from build123d import *

# Parameters (mm, degrees)
SKETCH1_W                                       = 50
SKETCH1_H                                       = 7.5
BOSS_EXTRUDE1_DEPTH                             = 5
FILLET1_R                                       = 2
SKETCH2_R                                       = 2.5
BOSS_EXTRUDE2_DEPTH                             = 3
CBORE_FOR_M3_SHCS1_D                            = 5.25
CBORE_FOR_M3_SHCS1_DEPTH                        = 4
CBORE_FOR_M3_SHCS1_CBORE_D                      = 6
CBORE_FOR_M3_SHCS1_CBORE_DEPTH                  = 0.5
CBORE_FOR_M3_SHCS1_TIP                          = 1.577259125
CSK_FOR_M3_FLAT_HEAD_MACHINE_SCREW1_D           = 3.4
CSK_FOR_M3_FLAT_HEAD_MACHINE_SCREW1_CSINK_D     = 6.3
CSK_FOR_M3_FLAT_HEAD_MACHINE_SCREW1_CSINK_ANGLE = 90
M3_CLEARANCE_HOLE1_D                            = 3.25
M3_CLEARANCE_HOLE1_DEPTH                        = 4
M3_CLEARANCE_HOLE1_TIP                          = 0.976398506


with BuildPart() as part:
    # Sketch1 → Boss-Extrude1 (new body)
    with BuildSketch(Plane(origin=(0, 0, 0), x_dir=(1, 0, 0), z_dir=(0, 1, 0))):
        with Locations((0, -8.75)):
            Rectangle(SKETCH1_W, SKETCH1_H)
        with BuildLine():
            Line((-25, 2.625), (-25, 5))
            ThreePointArc((-25, 5), (-30, 0), (-25, -5))
            Line((-25, -5), (-25, -2.625))
            ThreePointArc((-25, -2.625), (-27.625, 0), (-25, 2.625))
        make_face()
        with BuildLine():
            Line((25, 5), (-25, 5))
            Line((-25, 5), (-25, 2.625))
            ThreePointArc((-25, 2.625), (-23.143844699, 1.856155301), (-22.375, 0))
            ThreePointArc((-22.375, 0), (-23.143844699, -1.856155301), (-25, -2.625))
            Line((-25, -2.625), (-25, -5))
            Line((-25, -5), (25, -5))
            Line((25, -5), (25, -2.625))
            ThreePointArc((25, -2.625), (22.375, 0), (25, 2.625))
            Line((25, 2.625), (25, 5))
        make_face()
        with Locations((0, 8.75)):
            Rectangle(SKETCH1_W, SKETCH1_H)
        with BuildLine():
            ThreePointArc((25, -5), (30, 0), (25, 5))
            Line((25, 5), (25, 2.625))
            ThreePointArc((25, 2.625), (26.856155301, 1.856155301), (27.625, 0))
            ThreePointArc((27.625, 0), (26.856155301, -1.856155301), (25, -2.625))
            Line((25, -2.625), (25, -5))
        make_face()
        with BuildLine():
            ThreePointArc((-22.375, 0), (-23.143844699, 1.856155301), (-25, 2.625))
            Line((-25, 2.625), (-25, -2.625))
            ThreePointArc((-25, -2.625), (-23.143844699, -1.856155301), (-22.375, 0))
        make_face()
        with BuildLine():
            Line((-25, -2.625), (-25, 2.625))
            ThreePointArc((-25, 2.625), (-27.625, 0), (-25, -2.625))
        make_face()
        with BuildLine():
            ThreePointArc((27.625, 0), (26.856155301, 1.856155301), (25, 2.625))
            Line((25, 2.625), (25, -2.625))
            ThreePointArc((25, -2.625), (26.856155301, -1.856155301), (27.625, 0))
        make_face()
        with BuildLine():
            Line((25, -2.625), (25, 2.625))
            ThreePointArc((25, 2.625), (22.375, 0), (25, -2.625))
        make_face()
    extrude(amount=BOSS_EXTRUDE1_DEPTH)

    # Fillet1
    fillet1_edges = [part.edges().sort_by_distance(p)[0] for p in [
        (25, 2.5, 12.5),
        (-25, 2.5, 12.5),
        (-25, 2.5, 5),
        (-25, 2.5, -5),
        (-25, 2.5, -12.5),
        (25, 2.5, -12.5),
        (25, 2.5, -5),
        (25, 2.5, 5),
    ]]
    fillet(fillet1_edges, radius=FILLET1_R)

    # Sketch2 → Boss-Extrude2 (add)
    with BuildSketch(Plane.XZ):
        with Locations(Location((-14.75, 8.25, 0), (0, 0, 90))):
            Circle(SKETCH2_R)
        with Locations(Location((14.75, -8.25, 0), (0, 0, 90))):
            Circle(SKETCH2_R)
    extrude(amount=BOSS_EXTRUDE2_DEPTH)

    # CBORE for M3 SHCS1
    with Locations(Plane(origin=(0, 5, 0), x_dir=(1, 0, 0), z_dir=(0, 1, 0))):
        with Locations((-14.75, -8.25), (14.75, 8.25)):
            CounterBoreHole(CBORE_FOR_M3_SHCS1_D / 2, CBORE_FOR_M3_SHCS1_CBORE_D / 2, CBORE_FOR_M3_SHCS1_CBORE_DEPTH, depth=CBORE_FOR_M3_SHCS1_DEPTH)
            with Locations((0, 0, -(CBORE_FOR_M3_SHCS1_DEPTH + CBORE_FOR_M3_SHCS1_TIP / 2))):  # 118° drill point
                Cone(0, CBORE_FOR_M3_SHCS1_D / 2, CBORE_FOR_M3_SHCS1_TIP, mode=Mode.SUBTRACT)

    # CSK for M3 Flat Head Machine Screw1 (through all)
    with Locations(Plane.XZ):
        with Locations((-25, 0), (25, 0)):
            CounterSinkHole(CSK_FOR_M3_FLAT_HEAD_MACHINE_SCREW1_D / 2, CSK_FOR_M3_FLAT_HEAD_MACHINE_SCREW1_CSINK_D / 2, counter_sink_angle=CSK_FOR_M3_FLAT_HEAD_MACHINE_SCREW1_CSINK_ANGLE)

    # M3 Clearance Hole1
    with Locations(Plane.XZ.offset(3)):
        with Locations((-14.75, 8.25), (14.75, -8.25)):
            Hole(M3_CLEARANCE_HOLE1_D / 2, depth=M3_CLEARANCE_HOLE1_DEPTH)
            with Locations((0, 0, -(M3_CLEARANCE_HOLE1_DEPTH + M3_CLEARANCE_HOLE1_TIP / 2))):  # 118° drill point
                Cone(0, M3_CLEARANCE_HOLE1_D / 2, M3_CLEARANCE_HOLE1_TIP, mode=Mode.SUBTRACT)


solid = part.part
Source: CAD feature listing. Evaluate the final solid. Frame: model axes, mm. A direction names the side the tool comes from. Round coordinates to 2 decimals unless told otherwise and drop trailing zeros. Loops run counter-clockwise (first coordinate to the right, second up) from the corner with the lowest first, then second, coordinate; pieces in that order, holes last. Notation, with made-up numbers: M 42.5,-2 L 92.5,-2 A28 ccw 92.5,29 Z; hole C -33.5,-33.75 d10. An arc over 180 degrees is marked long. Return JSON: item names as keys, results as strings. Group by question number.
1. Reachability of faces 1 (the face through (-26.57, 3.25, -0.65)), 2 (the face through (-12.815, 2.726, 6.476)), 3 (the face through (-12.53, -1.48, 9.4)) from +Z, -Z, +X, -X, +Y, -Y: full face, straight path, thin tool, end or side. Return the list, or none.
2. Section query C-C on z = 0. Output: boundary loops of the cut face in (x, y).
3. Section query D-D on y = -2.25. Output: boundary loops of the cut face in (x, z) (3 decimals).
4. Section query B-B on z = 8.25. Output: boundary loops of the cut face in (x, y) (3 decimals), and give its area (3 significant figures).
5. Section query A-A on x = -14.75. Output: boundary loops of the cut face in (y, z) (3 decimals), and give its area (3 significant figures).
6. Pin query (flat end, axial travel): pin 1 (4.5 mm diameter, centred on x = -14.75, z = 8.25, fed in from -Y); pin 2 (1.1 mm diameter, centred on y = 3.5, z = 8.5, fed in from -X); pin 3 (4 mm diameter, centred on y = 3, z = -8, fed in from +X); pin 4 (3 mm diameter, centred on x = -14.75, z = 8.25, fed in from -Y). Return the tip coordinate at first contact, or that it passes through.
7. Mould query, pull axis X, two halves, no side actions, for faces 4 (the face through (24.4, 2.54, 11.93)), 5 (the face through (-25, 2, -9)), 6 (the face through (0, 5, 0)), 7 (the face through (16.685, 2.726, -10.024)). Classes: released by +X, released by -X, zero draft, split by the parting line, or undercut.
8. Material intervals for line 1 along X through (y, z) = (3.2, -8.25) (3 decimals); line 2 along X through (y, z) = (4.5, 0.25); line 3 along Z through (x, y) = (-14.75, 4.8), sorted ascending. Write a range as from..to.
Checks:
{
 "1": {"face 1": "+Y, -Y", "face 2": "+Y", "face 3": "-Y"},
 "2": {"outline": "M -30,0 L -28.15,0 L -26.7,1.45 L -26.7,5 L -30,5 Z; M -23.3,1.45 L -21.85,0 L 21.85,0 L 23.3,1.45 L 23.3,5 L -23.3,5 Z; M 26.7,1.45 L 28.15,0 L 30,0 L 30,5 L 26.7,5 Z"},
 "3": {"outline": "C -14.75,8.25 d5; C 14.75,-8.25 d5; hole C -14.75,8.25 d3.25; hole C 14.75,-8.25 d3.25"},
 "4": {"outline": "M -25,0 L -17.25,0 L -17.25,-3 L -16.375,-3 L -16.375,0.399 L -17.375,1 L -17.375,4.5 L -17.75,4.5 L -17.75,5 L -25,5 Z; M -13.125,-3 L -12.25,-3 L -12.25,0 L 25,0 L 25,5 L -11.75,5 L -11.75,4.5 L -12.125,4.5 L -12.125,1 L -13.125,0.399 Z", "area": "230 mm²"},
 "5": {"outline": "M -3,5.75 L 0,5.75 L 0,-12.5 L 5,-12.5 L 5,5.25 L 4.5,5.25 L 4.5,5.625 L 1,5.625 L 0.399,6.625 L -3,6.625 Z; M -3,9.875 L 0.399,9.875 L 1,10.875 L 4.5,10.875 L 4.5,11.25 L 5,11.25 L 5,12.5 L 0,12.5 L 0,10.75 L -3,10.75 Z", "area": "105 mm²"},
 "6": {"pin 1": "stops at y = -3", "pin 2": "stops at x = -25", "pin 3": "stops at x = 25.13", "pin 4": "passes through"},
 "7": {"face 4": "released by +X", "face 5": "released by -X", "face 6": "zero draft", "face 7": "undercut"},
 "8": {"line 1": "x = -25..12.125, 17.375..25", "line 2": "x = -29.99..-26.68, -23.32..23.32, 26.68..29.99", "line 3": "z = -12.5..5.25, 11.25..12.5"}
}
